Here's how the part is built. I have some questions about the finished solid (model axes, mm). A direction names the side the tool comes from. Round coordinates to 2 decimals unless told otherwise and drop trailing zeros. Write each loop counter-clockwise with the first axis right and the second up, starting at its lowest first coordinate (ties: lowest second). Pieces come first, ordered by that corner, then holes. Notation, with made-up numbers: M 28.5,3 L 38.5,3 A22 ccw 38.5,40 Z; hole C 43,-21.5 d10. An arc over 180 degrees is marked long. Use a Markdown table: item, result. Add a question column.
```python
from build123d import *

# Parameters (mm, degrees)
F0_W     = 254
F0_H     = 304.8
F1_DEPTH = 9.525
F2_R     = 9.52499
F4_DEPTH = 19.051


# Not quite as in the source:
# - a fillet or chamfer is up to 0.001 mm smaller than in the source, because OpenCascade refuses the exact size
# - a feature names something its author has since deleted; it is built from what else it names


with BuildPart() as f1:
    # F0 (on Right) → F1 (new body, symmetric)
    with BuildSketch(Plane.YZ):
        Rectangle(F0_W, F0_H)
    extrude(amount=F1_DEPTH, both=True)

    # F2 (radius 9.525 in the source; OpenCascade refuses exactly that, so slightly less here)
    f2_edges = [f1.edges().sort_by_distance(p)[0] for p in [
        (9.525, -127, 0),
        (-9.525, -127, 0),
    ]]
    fillet(f2_edges, radius=F2_R)

    # F3 (on face) → F4 (cut, through all)
    with BuildSketch(Plane.YZ.offset(9.525)):
        Polygon((107.95, 57.15), (127, 62.2544321158), (127, 128.2455678842), (107.95, 133.35), align=None)
        Polygon((127, -32.9955678842), (127, 32.9955678842), (107.95, 38.1), (107.95, -38.1), align=None)
        Polygon((127, -128.2455678842), (127, -62.2544321158), (107.95, -57.15), (107.95, -133.35), align=None)
    extrude(amount=-F4_DEPTH, mode=Mode.SUBTRACT)


solid = f1.part
```
Item 1: On a 3-axis mill with a long thin cutter (end or side, diameter ignored), from which of +Z, -Z, +X, -X, +Y, -Y can I reach the whole of each face in a straight line? I mean faces 4 (the face through (0.133, 117.342, -130.834)), 5 (the face through (0, -2, 152.4)). Say none if no direction works.
Item 2: For pin 1 Ø5 at (x, z) = (-0.5, -101.5) entering from +Y; pin 2 Ø2 at (x, z) = (2.5, -25) entering from -Y, each with a flat end and sliding along its axis, tell me the tip position at first contact or that it passes through.
Item 3: I need wall thicknesses on probe 1 along Y at (x, z) = (-0.25, 9.5); probe 2 along Y at (x, z) = (1, -113). Which ranges of each line are inside material? Lowest first, please. Write a range as from..to.
Item 4: If we mould it in two halves opening along Z, with no side actions, what happens to faces 1 (the face through (6.661, -124.284, 2.134)), 2 (the face through (0, -2, -152.4)), 3 (the face through (0, 107.95, 96))? For each: +Z half, -Z half, draft (parallel to the pull), parting line (faces both ways), or undercut.
Item 5: Imagine slicing it at A-A on x = 3.75. List the corners of the cut face in (y, z) for me.
The answers:
| question | item | result |
|---|---|---|
| 1 | face 4 | +X, -X |
| 1 | face 5 | +Z, +X, -X, +Y, -Y |
| 2 | pin 1 | y = 107.95 |
| 2 | pin 2 | y = -126.88 |
| 3 | probe 1 | -127..107.95 |
| 3 | probe 2 | -126.95..107.95 |
| 4 | face 1 | draft |
| 4 | face 2 | -Z half |
| 4 | face 3 | undercut |
| 5 | outline | M -126.23,-152.4 L 127,-152.4 L 127,-128.25 L 107.95,-133.35 L 107.95,-57.15 L 127,-62.25 L 127,-33 L 107.95,-38.1 L 107.95,38.1 L 127,33 L 127,62.25 L 107.95,57.15 L 107.95,133.35 L 127,128.25 L 127,152.4 L -126.23,152.4 Z |
